from build123d import *

# Parameters (mm, degrees)
F1_DEPTH = 1
F3_DEPTH = 1.5
F4_W     = 23
F4_H     = 5.8
F5_DEPTH = 2.5


with BuildPart() as f1:
    # F0 (on Top) → F1 (new body)
    with BuildSketch(Plane.XY):
        with BuildLine():
            ThreePointArc((0, 2), (0.585786, 0.585786), (2, 0))
            Line((2, 0), (55, 0))
            ThreePointArc((55, 0), (56.414214, 0.585786), (57, 2))
            Line((57, 2), (57, 20))
            Line((57, 20), (0, 20))
            Line((0, 20), (0, 2))
        make_face()
    extrude(amount=F1_DEPTH)

    # F2 (on face) → F3 (join)
    with BuildSketch(Plane.XY.offset(1)):
        with BuildLine():
            Line((54.75, 20), (2.25, 20))
            Line((2.25, 20), (2.25, 2))
            ThreePointArc((2.25, 2), (2.835786, 0.585786), (4.25, 0))
            Line((4.25, 0), (52.75, 0))
            ThreePointArc((52.75, 0), (54.164214, 0.585786), (54.75, 2))
            Line((54.75, 2), (54.75, 20))
        make_face()
    extrude(amount=F3_DEPTH)

    # F4 (on face) → F5 (cut, through all)
    with BuildSketch(Plane.XY):
        with Locations((20, 17.1)):
            Rectangle(F4_W, F4_H)
        Polygon((47.3, 20), (36, 20), (36, 17), (38, 17), (38, 15), (47.3, 15), align=None)
        with BuildLine():
            Line((42.5, 9.3), (32.5, 9.3))
            ThreePointArc((32.5, 9.3), (32.146447, 9.153553), (32, 8.8))
            Line((32, 8.8), (32, 0.8))
            ThreePointArc((32, 0.8), (32.146447, 0.446447), (32.5, 0.3))
            Line((32.5, 0.3), (42.5, 0.3))
            ThreePointArc((42.5, 0.3), (42.853553, 0.446447), (43, 0.8))
            Line((43, 0.8), (43, 8.8))
            ThreePointArc((43, 8.8), (42.853553, 9.153553), (42.5, 9.3))
        make_face()
    extrude(amount=F5_DEPTH, mode=Mode.SUBTRACT)


solid = f1.part
Verification items for the finished model (mm, model axes). A direction names the side the tool comes from. Coordinates: 2 decimals unless noted, no trailing zeros. Order: outer loops, then holes, each group sorted by start corner. A loop starts at its lowest first (then second) coordinate and runs counter-clockwise, first axis right, second up. Notation, with made-up numbers: M 59,7 L 77,7 A24 ccw 77,17 Z; hole C 46,60.25 d4. An arc over 180 degrees is marked long. Write each question's results on one line, items separated by ' | '.
1) Section check C-C on y = 18.75. Record the cut outline in (x, z), plus the area to 3 significant figures.
Solved:
outline: M 0,0 L 8.5,0 L 8.5,2.5 L 2.25,2.5 L 2.25,1 L 0,1 Z; M 31.5,0 L 36,0 L 36,2.5 L 31.5,2.5 Z; M 47.3,0 L 57,0 L 57,1 L 54.75,1 L 54.75,2.5 L 47.3,2.5 Z | area: 50.0 mm²
2) Access from +Z, -Z, +X, -X, +Y, -Y to the whole of each face (thin tool, end or side, straight path). Record for faces 1 (the face through (54.75, 11, 2)), 2 (the face through (31.5, 17, 1)), 3 (the face through (38, 9.3, 1)), 4 (the face through (2.25, 11, 2)), 5 (the face through (54.15, 0.57, 1.74)).
Solved:
face 1: +Z, +X, +Y, -Y | face 2: +Z, -Z, +Y | face 3: +Z, -Z | face 4: +Z, -X, +Y, -Y | face 5: +Z, +X, -Y
3) Gauge pin test, flat end, axial feed: pin 1 Ø1.3 at (x, y) = (55, 10) entering from +Z. Record the tip position at first contact, or that the pin passes through.
Solved:
pin 1: stops at z = 2.5
4) Section check D-D on y = 10. Record the cut outline in (x, z).
Solved:
outline: M 0,0 L 57,0 L 57,1 L 54.75,1 L 54.75,2.5 L 2.25,2.5 L 2.25,1 L 0,1 Z
5) Scan lines: line 1 along X through (y, z) = (16.75, 2.25); line 2 along X through (y, z) = (5, 1.2); line 3 along Y through (x, z) = (29.5, 1.35). Record each from-to range of solid material in increasing order. Write a range as [from, to].
Solved:
line 1: x = [2.25, 8.5], [31.5, 38], [47.3, 54.75] | line 2: x = [2.25, 32], [43, 54.75] | line 3: y = [0, 14.2]
6) Section check B-B on z = 1.4. Record the cut outline in (x, y).
Solved:
outline: M 2.25,2 A2 ccw 4.25,0 L 52.75,0 A2 ccw 54.75,2 L 54.75,20 L 47.3,20 L 47.3,15 L 38,15 L 38,17 L 36,17 L 36,20 L 31.5,20 L 31.5,14.2 L 8.5,14.2 L 8.5,20 L 2.25,20 Z; hole M 32,0.8 A0.5 ccw 32.5,0.3 L 42.5,0.3 A0.5 ccw 43,0.8 L 43,8.8 A0.5 ccw 42.5,9.3 L 32.5,9.3 A0.5 ccw 32,8.8 Z
7) Section check A-A on y = 3.5. Record the cut outline in (x, z).
Solved:
outline: M 0,0 L 32,0 L 32,2.5 L 2.25,2.5 L 2.25,1 L 0,1 Z; M 43,0 L 57,0 L 57,1 L 54.75,1 L 54.75,2.5 L 43,2.5 Z
8) Release check for a two-part mould opening along Y. For faces 6 (the face through (52, 20, 1)), 7 (the face through (43, 5, 1)), 8 (the face through (56.4, 0.57, 0.49)) record: pulls with the +Y half, pulls with the -Y half, needs draft (parallel to the pull), parting line crosses it, or undercut.
Solved:
face 6: pulls with the +Y half | face 7: undercut | face 8: pulls with the -Y half
